from build123d import *

# Parameters (mm, degrees)
SKETCH1_R           = 32.5
SKETCH1_R_2         = 0.889
SKETCH1_R_3         = 0.5335
BOSS_EXTRUDE1_DEPTH = 3
SKETCH2_W           = 45
SKETCH2_H           = 17
BOSS_EXTRUDE2_DEPTH = 5
LOFT1_START         = -19.5
LOFT1_DEPTH         = 17
FILLET2_R           = 10
CUT_EXTRUDE7_DEPTH  = 6.5
CUT_EXTRUDE8_DEPTH  = 9
SKETCH59_R          = 1.05
CUT_EXTRUDE9_DEPTH  = 6
SKETCH60_R          = 3.5
CUT_EXTRUDE10_DEPTH = 62.304245363
BOSS_EXTRUDE3_DEPTH = 11
CUT_EXTRUDE11_REACH = 53.415
SKETCH62_W          = 9.042987319
SKETCH62_H          = 2.5
SKETCH63_W          = 22
SKETCH63_H          = 5.75
CUT_EXTRUDE12_DEPTH = 10


# Read off the part's stored shape, not the designer's step: Loft1
with BuildPart() as part:
    # Sketch1 → Boss-Extrude1 (new body)
    with BuildSketch(Plane(origin=(0, 0, 0), x_dir=(1, 0, 0), z_dir=(0, 1, 0))):
        with Locations(Location((0, 0, 0), (0, 0, 270))):
            Circle(SKETCH1_R)
        with Locations(Location((0, 0, 0), (0, 0, 270))):
            Circle(SKETCH1_R_2, mode=Mode.SUBTRACT)
        with Locations(Location((-8.306, 0, 0), (0, 0, 270))):
            Circle(SKETCH1_R_3, mode=Mode.SUBTRACT)
        with Locations(Location((8.306, 0, 0), (0, 0, 90))):
            Circle(SKETCH1_R_3, mode=Mode.SUBTRACT)
    extrude(amount=BOSS_EXTRUDE1_DEPTH)

    # Sketch2 → Boss-Extrude2 (add)
    with BuildSketch(Plane(origin=(0, 3, 0), x_dir=(1, 0, 0), z_dir=(0, 1, 0))):
        with Locations((-2.5, 11)):
            Rectangle(SKETCH2_W, SKETCH2_H)
    extrude(amount=BOSS_EXTRUDE2_DEPTH)

    # Loft1 outline → Loft1 (add)
    with BuildSketch(Plane.XY.offset(LOFT1_START)):
        with BuildLine():
            Line((-25, 8), (20, 8))
            add(Edge.make_bspline(
                [(20, 8), (20.013119001, 12.366637273), (19.711715011, 23.342908392), (26.277458631, 32.792620463), (30.786821215, 37.0096)],
                knots=[0, 0, 0, 0, 0.412101617, 1, 1, 1, 1], degree=3))
            Line((30.786821215, 37.0096), (-19.558686419, 37.0096))
            Line((-19.558686419, 37.0096), (-25, 8))
        make_face()
    extrude(amount=LOFT1_DEPTH)

    # Fillet2
    fillet2_edges = [part.edges().sort_by_distance(p)[0] for p in [
        (30.786821215, 37.0096, -11),
        (-19.558686419, 37.0096, -11),
    ]]
    fillet(fillet2_edges, radius=FILLET2_R)

    # Sketch56 → Cut-Extrude7 (cut)
    with BuildSketch(Plane(origin=(0, 0, -19.5), x_dir=(-1, 0, 0), z_dir=(0, 0, -1))):
        with BuildLine():
            Line((11.259989716, 35.0096), (-12.262162003, 35.0096))
            ThreePointArc((-12.262162003, 35.0096), (-18.800326154, 31.619633572), (-19.797451062, 24.322702384))
            add(Edge.make_bspline(
                [(-19.797451062, 24.322702384), (-19.33456189, 23.024549565), (-18.970633179, 21.699807372), (-18.444923303, 18.9960086), (-18.278988003, 17.628977113), (-18.070720499, 14.883614823), (-18.028473243, 13.506968306), (-17.995025378, 10.755326884), (-18.004134147, 9.379048249), (-18, 8.003004365)],
                knots=[0, 0, 0, 0, 0.25, 0.25, 0.5, 0.5, 0.75, 0.75, 1, 1, 1, 1], degree=3))
            Line((-18, 8.003004365), (-18, 5))
            Line((-18, 5), (23, 5))
            Line((23, 5), (23, 7.814051971))
            Line((23, 7.814051971), (19.122868337, 28.484435511))
            ThreePointArc((19.122868337, 28.484435511), (16.368870019, 33.165844151), (11.259989716, 35.0096))
        make_face()
    extrude(amount=-CUT_EXTRUDE7_DEPTH, mode=Mode.SUBTRACT)

    # Sketch57 → Cut-Extrude8 (cut)
    with BuildSketch(Plane(origin=(0, 0, -13), x_dir=(-1, 0, 0), z_dir=(0, 0, -1))):
        Polygon((-6.147589592, 30.253616288), (-12.539757722, 19.62816634), (6.997359924, 7.874824939), (13.389528054, 18.500274887), align=None)
    extrude(amount=-CUT_EXTRUDE8_DEPTH, mode=Mode.SUBTRACT)

    # Sketch59 → Cut-Extrude9 (cut)
    with BuildSketch(Plane(origin=(0, 0, -13), x_dir=(-1, 0, 0), z_dir=(0, 0, -1))):
        with Locations((-11.850080197, 26.448721296)):
            Circle(SKETCH59_R)
        with Locations((12.699850529, 11.679719931)):
            Circle(SKETCH59_R)
    extrude(amount=-CUT_EXTRUDE9_DEPTH, mode=Mode.SUBTRACT)

    # Sketch60 → Cut-Extrude10 (cut, through all)
    with BuildSketch(Plane(origin=(0, 0, -4), x_dir=(-1, 0, 0), z_dir=(0, 0, -1))):
        with Locations((-4.287675332, 22.191003874)):
            Circle(SKETCH60_R)
    extrude(amount=-CUT_EXTRUDE10_DEPTH, mode=Mode.SUBTRACT)

    # Sketch61 → Boss-Extrude3 (add)
    with BuildSketch(Plane.XY.offset(-2.5)):
        Polygon((-25, 3), (-15.957012681, 3), (-15.957012681, 4.875346451), (-22.634257591, 4.875346451), (-22.634257591, 8.517700202), (-22.634257591, 11.401095106), (-19.020402646, 11.401095106), (-19.020402646, 7.370992949), (-15.957012681, 7.370992949), (-15.957012681, 13.965550524), (-23.881045203, 13.965550524), (-25, 8), align=None)
    extrude(amount=BOSS_EXTRUDE3_DEPTH)

    # Cut-Extrude11: up to this face of the body (flat: up to its plane)
    cut_extrude11_end = Plane(part.part.faces().sort_by_distance((1.612350985, 3, 3.31348115))[0])
    # Sketch62 → Cut-Extrude11 (cut, up to the picked face)
    with BuildSketch(Plane(origin=(0, 13.965550524, 0), x_dir=(1, 0, 0), z_dir=(0, 1, 0)), mode=Mode.PRIVATE) as cut_extrude11_sk1:
        with Locations((-20.478506341, 1.25)):
            Rectangle(SKETCH62_W, SKETCH62_H)
    cut_extrude11_tool1 = split(extrude(cut_extrude11_sk1.sketch, amount=-CUT_EXTRUDE11_REACH, mode=Mode.PRIVATE), bisect_by=cut_extrude11_end, keep=Keep.BOTH, mode=Mode.PRIVATE)
    add(cut_extrude11_tool1.solids().sort_by(Axis((-20.478506, 13.965551, -1.25), (0, -1, 0)))[0], mode=Mode.SUBTRACT)

    # Sketch63 → Cut-Extrude12 (cut)
    with BuildSketch(Plane(origin=(0, 3, 0), x_dir=(1, 0, 0), z_dir=(0, 1, 0))):
        with Locations((-0.259989716, 24.466538137)):
            Rectangle(SKETCH63_W, SKETCH63_H)
    extrude(amount=-CUT_EXTRUDE12_DEPTH, mode=Mode.SUBTRACT)


solid = part.part
Work out the finished part from the listing and answer in its coordinate system (mm). A direction names the side the tool comes from. Coordinates: 2 decimals unless noted, no trailing zeros. Loops run counter-clockwise (first coordinate to the right, second up) from the corner with the lowest first, then second, coordinate; pieces in that order, holes last. Notation, with made-up numbers: (41, 30.5) -> (79, 30.5) arc R22 cw to (79, 37.5) -> close; hole circle Ø8 at (5.5, -39). An arc over 180 degrees is marked (long way). Answer as CSV lines item,"result".
1) Flat-ended cylindrical pins translate along their axes: pin 1 (0.9 mm diameter, centred on y = 1.5, z = -24.5, fed in from -X); pin 2 (1.7 mm diameter, centred on x = 8.306, z = 0, fed in from +Y); pin 3 (6 mm diameter, centred on x = 4.5, y = 5.5, fed in from +Z); pin 4 (5 mm diameter, centred on y = 7, z = 19.5, fed in from -X). Find the tip coordinate at first contact, or state that the pin passes through.
A:
pin 1,"stops at x = -21.86"
pin 2,"stops at y = 3"
pin 3,"stops at z = 32.38"
pin 4,"passes through"
2) The part is cut by section A-A (z = 27). Give the vertices of the cut face in (x, y).
A:
outline,"(-18.09, 0) -> (18.09, 0) -> (18.09, 3) -> (-18.09, 3) -> close"
3) For faces 1 (the face through (-18.5, 8.6, 0)), 2 (the face through (-15.957, 4, 4)), 3 (the face through (-11.26, 2, -24)), 4 (the face through (-21.09, 18, -16.3)), determine the directions among +Z, -Z, +X, -X, +Y, -Y from which every point of the face is accessible in a straight line to the end or side of a thin tool.
A:
face 1,"+X, -X, +Y"
face 2,"+Z, +X, +Y"
face 3,"+Y, -Y"
face 4,"-Z"
4) For a pull along X with two mould halves and no side action, classify faces 5 (the face through (-22.634, 8, 4)), 6 (the face through (-24.433, 11.025, 4.19)), 7 (the face through (0, 0, 7)) as released by +X, released by -X, zero draft, split by the parting line, or undercut.
A:
face 5,"undercut"
face 6,"released by -X"
face 7,"zero draft"
5) Straight lines are drawn through the part: probe 1 along X at (y, z) = (1.6, 0); probe 2 along Y at (x, z) = (8, -14); probe 3 along Z at (x, y) = (16.5, 12). For each, find the intervals that lie inside material, in ascending order.
A:
probe 1,"x = -32.5 to -8.84, -7.77 to -0.89, 0.89 to 7.77, 8.84 to 32.5"
probe 2,"y = 0 to 5, 35.01 to 37.01"
probe 3,"z = -13 to -2.5"
